Autodesk Inventor part; units mm, degrees
ref_plane "YZ Plane" through (0, 0, 0) normal (1, 0, 0) x (0, 1, 0)
ref_plane "XZ Plane" through (0, 0, 0) normal (0, 1, 0) x (-1, 0, 0)
sketch "Skizze8" plane through (0, 0, 0) normal (0, 0, 1) x (1, 0, 0)
  line L0 (0, 0) -> (0, 22.5)
  line L1 (0, 22.5) -> (21.65, 22.5)
  line L2 (21.65, 22.5) -> (21.65, 29)
  line L3 (21.65, 29) -> (37.65, 29)
  line L4 (37.65, 29) -> (37.65, 22.5)
  line L5 (37.65, 22.5) -> (59.3, 22.5)
  line L6 (59.3, 22.5) -> (59.3, 16)
  line L7 (59.3, 16) -> (126.3, 16)
  line L8 (126.3, 16) -> (126.3, 0)
  line L9 (126.3, 0) -> (0, 0)
  line L10 (-25.26, 0) -> (151.56, 0)
revolve "Umdrehung7" add sketch "Skizze8" angle 360 about axis through (-10, 0, 0) along (1, 0, 0)
sketch "Skizze9" plane through (0, 0, 0) normal (0, 0, 1) x (1, 0, 0)
  line L0 (3.8, 21.25) -> (5.65, 21.25)
  line L1 (5.65, 21.25) -> (5.65, 22.5)
  line L2 (5.65, 22.5) -> (3.8, 22.5)
  line L3 (3.8, 22.5) -> (3.8, 21.25)
  line L4 (-25.26, 0) -> (151.56, 0)
revolve "Umdrehung8" cut sketch "Skizze9" angle 360 about axis through (-10, 0, 0) along (1, 0, 0)
sketch "Skizze10" plane through (0, 0, 0) normal (0, 0, 1) x (1, 0, 0)
  line L0 (21.65, 24.5) -> (21.85, 23.7536)
  line L1 (20.2696, 22.2) -> (19.15, 22.5)
  line L2 (19.15, 22.5) -> (19.15, 24.5)
  line L3 (19.15, 24.5) -> (21.65, 24.5)
  arc A0 (20.2696, 22.2) -> (21.85, 23.7536) centre (20.7794, 23.262) ccw
  line L4 (-25.26, 0) -> (151.56, 0)
revolve "Umdrehung9" cut sketch "Skizze10" angle 360 about axis through (-10, 0, 0) along (1, 0, 0)
sketch "Skizze11" plane through (0, 0, 0) normal (0, 0, 1) x (1, 0, 0)
  line L0 (55.5, 21.25) -> (53.65, 21.25)
  line L1 (53.65, 21.25) -> (53.65, 22.5)
  line L2 (53.65, 22.5) -> (55.5, 22.5)
  line L3 (55.5, 22.5) -> (55.5, 21.25)
  line L4 (-25.26, 0) -> (151.56, 0)
revolve "Umdrehung10" cut sketch "Skizze11" angle 360 about axis through (-10, 0, 0) along (1, 0, 0)
sketch "Skizze12" plane through (0, 0, 0) normal (0, 0, 1) x (1, 0, 0)
  line L0 (37.65, 24.5) -> (37.45, 23.7536)
  line L1 (39.0304, 22.2) -> (40.15, 22.5)
  line L2 (40.15, 22.5) -> (40.15, 24.5)
  line L3 (40.15, 24.5) -> (37.65, 24.5)
  arc A0 (37.45, 23.7536) -> (39.0304, 22.2) centre (38.5206, 23.262) ccw
  line L4 (-25.26, 0) -> (151.56, 0)
revolve "Umdrehung11" cut sketch "Skizze12" angle 360 about axis through (-10, 0, 0) along (1, 0, 0)
ref_plane "Arbeitsebene2" through (0, 0, 16) normal (0, 0, 1) x (1, 0, 0)
sketch "Skizze13" plane through (0, 0, 16) normal (0, 0, 1) x (1, 0, 0)
  line L0 (64.8, 0) -> (120.8, 0) construction
  line L1 (69.8, -5) -> (115.8, -5)
  line L2 (115.8, 5) -> (69.8, 5)
  arc A0 (69.8, 5) -> (69.8, -5) centre (69.8, 0) ccw
  arc A1 (115.8, -5) -> (115.8, 5) centre (115.8, 0) ccw
  point P0 (92.8, 0)
extrude "Extrusion2" cut sketch "Skizze13" against normal blind 5
sketch "Skizze14" plane through (0, 0, 0) normal (0, 0, 1) x (1, 0, 0)
  line L0 (59.3, 18) -> (59.1, 17.2536)
  line L1 (60.6804, 15.7) -> (61.8, 16)
  line L2 (61.8, 16) -> (61.8, 18)
  line L3 (61.8, 18) -> (59.3, 18)
  arc A0 (59.1, 17.2536) -> (60.6804, 15.7) centre (60.1706, 16.762) ccw
  line L4 (-25.26, 0) -> (151.56, 0)
revolve "Umdrehung12" cut sketch "Skizze14" angle 360 about axis through (-10, 0, 0) along (1, 0, 0)
properties part number "1"
Here's how the part is built. I have some questions about the finished solid (model axes, mm). A direction names the side the tool comes from. Coordinates: 2 decimals unless noted, no trailing zeros. Order: outer loops, then holes, each group sorted by start corner. A loop starts at its lowest first (then second) coordinate and runs counter-clockwise, first axis right, second up.
Item 1: If we mould it in two halves opening along X, with no side actions, what happens to faces 1 (the face through (120.8, -0.1, 13.5)), 2 (the face through (59.3, -10.1, 15.1)), 3 (the face through (46.994, 10.382, -19.961)), 4 (the face through (5.65, -13, -17))? For each: +X half, -X half, draft (parallel to the pull), parting line (faces both ways), or undercut.
Result sheet:
face 1: undercut
face 2: +X half
face 3: draft
face 4: undercut
Item 2: For P1, Ø4, axis at x = 25, z = 8, coming from the -Y side; P2, Ø6, axis at x = 112, y = 17.5, coming from the +Z side; P3, Ø1, axis at x = 78, y = -5.5, coming from the -Z side, each with a flat end and sliding along its axis, tell me the tip position at first contact or that it passes through.
Result sheet:
P1: stops at y = -28.37
P2: stops at z = 6.76
P3: stops at z = -15.2
Item 3: If we section it at A-A on x = 11: List the corners of the cut face in (y, z) for me.
Result sheet:
outline: circle Ø45 at (0, 0)
Item 4: I need wall thicknesses on line 1 (X direction, y = -8, z = 25); line 2 (X direction, y = 0, z = 18); line 3 (Y direction, x = 36.5, z = -0.5). Which ranges of each line are inside material? Lowest first, please.
Result sheet:
line 1: x = 21.65 to 37.65
line 2: x = 0 to 59.3
line 3: y = -29 to 29
Item 5: For faces 5 (the face through (64.8, 0.1, 13.5)), 6 (the face through (57.427, 10.382, -19.961)), 7 (the face through (12.494, 10.382, -19.961)), 8 (the face through (53.65, -13, -17)), which set-ups out of +Z, -Z, +X, -X, +Y, -Y let a thin tool reach every point of the face, with its end or its side?
Result sheet:
face 5: +Z
face 6: +X
face 7: -X
face 8: none
